Source: CAD feature listing. Evaluate the final solid. Frame: model axes, mm. A direction names the side the tool comes from. Give positions to 0.01 mm unless a question says otherwise; leave off trailing zeros. Loops run counter-clockwise (first coordinate to the right, second up) from the corner with the lowest first, then second, coordinate; pieces in that order, holes last. Notation, with made-up numbers: M 58.5,-20.75 L 62.5,-20.75 A19 cw 62.5,-4.75 Z; hole C 39.5,-6.75 d1. An arc over 180 degrees is marked long. Answer in a Markdown table with one row per item.
```python
from build123d import *

# Parameters (mm, degrees)
BOSS_EXTRUDE1_DEPTH     = 6
SKETCH2_R               = 2
CUT_EXTRUDE1_DEPTH      = 31.894983412
CHAMFER1_SIZE           = 2
DIAMETER_HOLE1_D        = 4.5
CUT_EXTRUDE2_DEPTH      = 29.151376521
CUT_EXTRUDE2_DEPTH_BACK = 29.151376521
SKETCH5_W               = 6
SKETCH5_H               = 18.5


with BuildPart() as part:
    # Sketch1 → Boss-Extrude1 (new, symmetric)
    with BuildSketch(Plane(origin=(0, 0, 0), x_dir=(0, 0, -1), z_dir=(1, 0, 0))):
        Polygon((-12.5, 0), (12.5, 0), (12.5, 5), (4.5, 5), (4.5, 24.5), (-4.5, 24.5), (-4.5, 5), (-12.5, 5), align=None)
    extrude(amount=BOSS_EXTRUDE1_DEPTH, both=True)

    # Sketch2 → Cut-Extrude1 (cut, through all)
    with BuildSketch(Plane(origin=(6, 0, -2), x_dir=(0, 0, 1), z_dir=(-1, 0, 0))):
        with Locations((2, 20)):
            Circle(SKETCH2_R)
    extrude(amount=CUT_EXTRUDE1_DEPTH, mode=Mode.SUBTRACT)

    # Chamfer1
    chamfer1_edges = [part.edges().sort_by_distance(p)[0] for p in [
        (0, 24.5, 4.5),
        (0, 24.5, -4.5),
    ]]
    chamfer(chamfer1_edges, length=CHAMFER1_SIZE)

    # Diameter Hole1 (through all)
    with Locations(Plane(origin=(5.400260834, 5, -6.193239857), x_dir=(-1, 0, 0), z_dir=(0, 1, 0))):
        with Locations((5.400260834, 15.193239857), (5.400260834, -2.806760143)):
            Hole(DIAMETER_HOLE1_D / 2)

    # Sketch5 → Cut-Extrude2 (cut, two sides: drawn at the far end of the back side and taken through both)
    with BuildSketch(Plane.XY.offset(-CUT_EXTRUDE2_DEPTH_BACK)):
        with Locations((0, 15.25)):
            Rectangle(SKETCH5_W, SKETCH5_H)
    extrude(amount=CUT_EXTRUDE2_DEPTH + CUT_EXTRUDE2_DEPTH_BACK, mode=Mode.SUBTRACT)


solid = part.part
```
Q1. Section query B-B (x = 0). Output: boundary loops of the cut face in (y, z).
Values follow:
| item | result |
|---|---|
| outline | M 0,-12.5 L 5,-12.5 L 5,-11.25 L 0,-11.25 Z; M 0,-6.75 L 5,-6.75 L 5,-4.5 L 6,-4.5 L 6,4.5 L 5,4.5 L 5,6.75 L 0,6.75 Z; M 0,11.25 L 5,11.25 L 5,12.5 L 0,12.5 Z |
Q2. Section query A-A (z = -9). Output: boundary loops of the cut face in (x, y).
Values follow:
| item | result |
|---|---|
| outline | M -6,0 L -2.25,0 L -2.25,5 L -6,5 Z; M 2.25,0 L 6,0 L 6,5 L 2.25,5 Z |
Q3. Section query D-D (y = 16). Output: boundary loops of the cut face in (x, z), plus the area to 3 significant figures.
Values follow:
| item | result |
|---|---|
| outline | M -6,-4.5 L -3,-4.5 L -3,4.5 L -6,4.5 Z; M 3,-4.5 L 6,-4.5 L 6,4.5 L 3,4.5 Z |
| area | 54.0 mm^2 |
Q4. Section query C-C (y = 20). Output: boundary loops of the cut face in (x, z).
Values follow:
| item | result |
|---|---|
| outline | M -6,-4.5 L -3,-4.5 L -3,-2 L -6,-2 Z; M -6,2 L -3,2 L -3,4.5 L -6,4.5 Z; M 3,-4.5 L 6,-4.5 L 6,-2 L 3,-2 Z; M 3,2 L 6,2 L 6,4.5 L 3,4.5 Z |
Q5. Mould query, pull axis X, two halves, no side actions, for faces 6 (the flat face through (3, 15, 0)), 7 (the flat face through (-5, 24, 3)), 8 (the flat face through (6, 10, 0)). Classes: +X half, -X half, draft (parallel to the pull), parting line (faces both ways), or undercut.
Values follow:
| item | result |
|---|---|
| face 6 | undercut |
| face 7 | draft |
| face 8 | +X half |
Q6. Contact query for flat-ended pins moving along their axis: pin 1 Ø4 at (x, z) = (2.5, 10) entering from +Y; pin 2 Ø6 at (x, y) = (-0.5, 16) entering from +Z. Output: stop coordinate, or through.
Values follow:
| item | result |
|---|---|
| pin 1 | y = 5 |
| pin 2 | z = 4.5 |
Q7. Reachability of faces 1 (the flat face through (5, 24.5, 0)), 2 (the flat face through (1.4, 5, -6.8)), 3 (the flat face through (4, 14, 4.5)), 4 (the cylindrical face through (-0.29, 2.47, 11.23)), 5 (the flat face through (0, 6, 0)) from +Z, -Z, +X, -X, +Y, -Y: full face, straight path, thin tool, end or side. Return the list, or none.
Values follow:
| item | result |
|---|---|
| face 1 | +Z, -Z, +X, -X, +Y |
| face 2 | -Z, +X, -X, +Y |
| face 3 | +Z, +X, -X, +Y |
| face 4 | +Y, -Y |
| face 5 | +Z, -Z, +Y |
Q8. Ray query, probe 1 along Z at (x, y) = (0, 2.85); probe 2 along Z at (x, y) = (4.7, 20); probe 3 along X at (y, z) = (14.75, 2). Return the intervals inside material, ascending. Write a range as from..to.
Values follow:
| item | result |
|---|---|
| probe 1 | -12.5..-11.25, -6.75..6.75, 11.25..12.5 |
| probe 2 | -4.5..-2, 2..4.5 |
| probe 3 | -6..-3, 3..6 |
